Source: CAD feature listing. Evaluate the final solid. Frame: model axes, mm. A direction names the side the tool comes from. Give positions to 0.01 mm unless a question says otherwise; leave off trailing zeros. Order: outer loops, then holes, each group sorted by start corner. A loop starts at its lowest first (then second) coordinate and runs counter-clockwise, first axis right, second up. Notation, with made-up numbers: M 29.25,-34 L 86.25,-34 A32 ccw 86.25,2 Z; hole C -27,-26.75 d3. An arc over 180 degrees is marked long. Return JSON: item names as keys, results as strings.
from build123d import *

# Parameters (mm, degrees)
SKETCH003_R     = 8.25
PAD_DEPTH       = 6
THICKNESS_T     = -0.5
SKETCH004_W     = 10
SKETCH004_H     = 9.446465
POCKET_DEPTH    = 2
SKETCH005_W     = 1.5
SKETCH005_H     = 1.5
POCKET001_DEPTH = 1.5
SKETCH006_W     = 0.5
SKETCH006_H     = 1.5
PAD001_DEPTH    = 1.5
SKETCH007_W     = 1.5
SKETCH007_H     = 0.5
PAD002_DEPTH    = 1.75


with BuildPart() as part:
    # Sketch003 → Pad (new body)
    with BuildSketch(Plane.XY):
        Circle(SKETCH003_R)
    extrude(amount=PAD_DEPTH)

    # Thickness
    thickness_openings = [part.faces().sort_by_distance(p)[0] for p in [
        (0, 0, 6),
    ]]
    offset(amount=THICKNESS_T, openings=thickness_openings)

    # Sketch004 (on DatumPlane) → Pocket (cut)
    with BuildSketch(Plane.XY.offset(6)):
        with Locations((0, -4.723232)):
            Rectangle(SKETCH004_W, SKETCH004_H)
    extrude(amount=-POCKET_DEPTH, mode=Mode.SUBTRACT)

    # Sketch005 (on DatumPlane) → Pocket001 (cut)
    with BuildSketch(Plane.YZ.offset(8.25)):
        with Locations((0, 0.75)):
            Rectangle(SKETCH005_W, SKETCH005_H)
    extrude(amount=-POCKET001_DEPTH, mode=Mode.SUBTRACT)

    # Sketch006 (on DatumPlane) → Pad001 (join)
    with BuildSketch(Plane.XY.offset(0.5)):
        with Locations((6.5, 0)):
            Rectangle(SKETCH006_W, SKETCH006_H)
    extrude(amount=PAD001_DEPTH)

    # Sketch007 (on DatumPlane) → Pad002 (join)
    with BuildSketch(Plane.YZ.offset(6.25)):
        with Locations((0, 1.75)):
            Rectangle(SKETCH007_W, SKETCH007_H)
    extrude(amount=PAD002_DEPTH)


solid = part.part
1. Section query A-A (z = 1.25). Return loops of the section in (x, y).
Evaluation:
{"outline": "M 6.25,-0.75 L 6.75,-0.75 L 6.75,0.75 L 6.25,0.75 Z; M 7.71,-0.75 A7.75 cw long 7.71,0.75 L 8.22,0.75 A8.25 ccw long 8.22,-0.75 Z"}
2. Section query B-B (x = 0). Return loops of the section in (y, z), then the cut area to 4 significant figures.
Evaluation:
{"outline": "M -8.25,0 L 8.25,0 L 8.25,6 L 7.75,6 L 7.75,0.5 L -7.75,0.5 L -7.75,4 L -8.25,4 Z", "area": "12.75 mm^2"}
3. Section query D-D (z = 2.4). Return loops of the section in (x, y).
Evaluation:
{"outline": "C 0,0 d16.5; hole C 0,0 d15.5"}
4. Draft query along X for faces 1 (the face through (6.75, 0, 1)), 2 (the face through (6.25, 0, 1)), 3 (the face through (8, 0.75, 1)). Return one class per face: pulls with the +X half, pulls with the -X half, needs draft (parallel to the pull), parting line crosses it, or undercut.
Evaluation:
{"face 1": "pulls with the +X half", "face 2": "undercut", "face 3": "needs draft"}
5. Section query C-C (y = 4.5). Return loops of the section in (x, z), then the cut area to 3 significant figures.
Evaluation:
{"outline": "M -6.91,0 L 6.91,0 L 6.91,6 L 6.31,6 L 6.31,0.5 L -6.31,0.5 L -6.31,6 L -6.91,6 Z", "area": "13.6 mm^2"}
6. Ray query, probe 1 along X at (y, z) = (-0.25, 4); probe 2 along Z at (x, y) = (-4.5, -3.25). Return the intervals inside material, ascending.
Evaluation:
{"probe 1": "x = -8.25 to -7.75, 7.75 to 8.25", "probe 2": "z = 0 to 0.5"}
7. Set-up query: faces 4 (the face through (6.6, 0.75, 1.4)), 5 (the face through (8, -0.75, 1)), 6 (the face through (-2.5, 7.5, 6)). Return all of +Z, -Z, +X, -X, +Y, -Y with unobstructed straight access to the full face (end or side cutting, diameter ignored); none if empty.
Evaluation:
{"face 4": "+Z", "face 5": "-Z, +X", "face 6": "+Z, +X, -X, +Y, -Y"}
8. First-contact query: pin 1 (1 mm diameter, centred on y = 3.5, z = 4, fed in from +X); pin 2 (2.5 mm diameter, centred on x = 0, y = -7, fed in from +Z); pin 3 (1.6 mm diameter, centred on x = 7, z = 1, fed in from -Y). Flat tips, straight axial feed; report the tip coordinate or a pass-through.
Evaluation:
{"pin 1": "stops at x = 7.69", "pin 2": "stops at z = 4", "pin 3": "stops at y = -5.44"}
